Geometry check sheet. Reference: the model listing, model coordinates, mm. Round coordinates to 2 decimals unless told otherwise and drop trailing zeros. Loops run counter-clockwise (first coordinate to the right, second up) from the corner with the lowest first, then second, coordinate; pieces in that order, holes last. Notation, with made-up numbers: M 69.25,64 L 85.25,64 A20 ccw 85.25,82 Z; hole C 65,35 d1. An arc over 180 degrees is marked long. Use one line per item in the form item = value. Start each with the question number.
1. Cross-section at B-B (x = 1221). Record the boundary of the cut face in (y, z).
2. Material ranges on line 1 (X direction, y = -903, z = 877.5); line 2 (Z direction, x = 2035.5, y = -876); line 3 (Y direction, x = 1590, z = 857), recorded low to high.
3. Cross-section at A-A (y = -872). Record the boundary of the cut face in (x, z), then the cut area to 3 significant figures.
4. Go/stop test with flat-tipped pins: pin 1 (5 mm diameter, centred on x = 647, y = -884, fed in from +Z); pin 2 (15.5 mm diameter, centred on x = 2454, z = 881.5, fed in from +Y); pin 3 (6 mm diameter, centred on x = 1710.5, z = 875.5, fed in from +Y); pin 4 (11 mm diameter, centred on x = 302, z = 879, fed in from -Y). Record where each tip stops, or that it passes through.
5. Draft check along X on faces 1 (the flat face through (1669, -879, 871.607)), 2 (the flat face through (308, -880, 885.557)), 3 (the flat face through (194.955, -879, 847)). Enter one of: pulls with the +X half, pulls with the -X half, needs draft (parallel to the pull), parting line crosses it, or undercut.
```python
from build123d import *

# Parameters (mm, degrees)
SKETCH014_W  = 2440
SKETCH014_H  = 48
PAD014_DEPTH = 70
SKETCH019_W  = 45
SKETCH019_H  = 70
PAD019_DEPTH = 13.95
SKETCH020_W  = 48
SKETCH020_H  = 70
PAD020_DEPTH = 13.95


with BuildPart() as part:
    # Sketch014 → Pad014 (new body)
    with BuildSketch(Plane.XZ):
        with Locations((1414.96, 859)):
            Rectangle(SKETCH014_W, SKETCH014_H)
    extrude(amount=PAD014_DEPTH)

    # Sketch019 (on Face1 of Pad014) → Pad019 (join)
    with BuildSketch(Plane(origin=(0, 0, 883), x_dir=(-1, 0, 0), z_dir=(0, 0, 1))):
        with Locations((-2449.118553, 35.037096)):
            Rectangle(SKETCH019_W, SKETCH019_H)
    extrude(amount=PAD019_DEPTH)

    # Sketch020 (on Face1 of Pad019) → Pad020 (join)
    with BuildSketch(Plane(origin=(0, 0, 883), x_dir=(-1, 0, 0), z_dir=(0, 0, 1))):
        with Locations((-308.031693, 34.93343)):
            Rectangle(SKETCH020_W, SKETCH020_H)
    extrude(amount=PAD020_DEPTH)


with BuildPart() as part_1:
    # Body011 placement: moved
    add(part.part.moved(Location((-0.005029, -844.254652, -11.393262))))


solid = part_1.part
```
Reported:
q1.outline = M -914.25,823.61 L -844.25,823.61 L -844.25,871.61 L -914.25,871.61 Z
q2.line_1 = 284.03 to 332.03, 2426.61 to 2471.61
q2.line_2 = 823.61 to 871.61
q2.line_3 = -914.25 to -844.25
q3.outline = M 194.95,823.61 L 2634.95,823.61 L 2634.95,871.61 L 2471.61,871.61 L 2471.61,885.56 L 2426.61,885.56 L 2426.61,871.61 L 332.03,871.61 L 332.03,885.56 L 284.03,885.56 L 284.03,871.61 L 194.95,871.61 Z
q3.area = 118,000 mm²
q4.pin_1 = 871.61
q4.pin_2 = -844.29
q4.pin_3 = through
q4.pin_4 = -914.19
q5.face_1 = undercut
q5.face_2 = needs draft
q5.face_3 = pulls with the -X half
